from build123d import *

# Parameters (mm, degrees)
F0_R     = 1.5
F1_DEPTH = 2
F0_W     = 15.1
F0_H     = 20
F2_DEPTH = 7.7
F3_R     = 1


with BuildPart() as f1:
    # F0 (on Top) → F1 (new body)
    with BuildSketch(Plane.XY):
        with BuildLine():
            Line((-7.55, 10), (7.55, 10))
            Line((7.55, 10), (5.552786, 13.994427))
            ThreePointArc((5.552786, 13.994427), (4.815394, 14.801302), (3.763932, 15.1))
            Line((3.763932, 15.1), (-3.763932, 15.1))
            ThreePointArc((-3.763932, 15.1), (-4.815394, 14.801302), (-5.552786, 13.994427))
            Line((-5.552786, 13.994427), (-7.55, 10))
        make_face()
        with Locations((0, 12)):
            Circle(F0_R, mode=Mode.SUBTRACT)
    extrude(amount=F1_DEPTH)

    # F0 (on Top) → F2 (join)
    with BuildSketch(Plane.XY):
        Rectangle(F0_W, F0_H)
    extrude(amount=F2_DEPTH)

    # F3
    f3_edges = [f1.edges().sort_by_distance(p)[0] for p in [
        (0, -10, 7.7),
        (7.55, 0, 7.7),
        (0, 10, 7.7),
        (-7.55, 0, 7.7),
    ]]
    fillet(f3_edges, radius=F3_R)


solid = f1.part
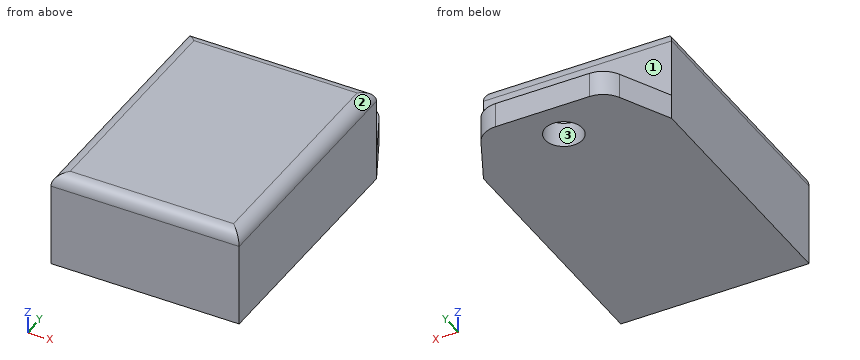
The listing builds one solid part. Answer for the finished solid, in the listing's coordinates (mm). Face numbers are marked on the shaded views. Coordinates: 2 decimals unless noted, no trailing zeros. Loops run counter-clockwise (first coordinate to the right, second up) from the corner with the lowest first, then second, coordinate; pieces in that order, holes last.
1) Find section C-C on z = 1. Write down the section's boundary in (x, y), then the cut area to 3 significant figures.
2) Determine the mould class of the marked faces 1, 2 and 3 for opening direction X: pulls with the +X half, pulls with the -X half, needs draft (parallel to the pull), parting line crosses it, or undercut.
3) Find section A-A on y = 12. Write down the section's boundary in (x, z).
4) Find section B-B on x = 0. Write down the section's boundary in (y, z).
5) Find the intervals of material crossed by L1, parallel to Y at x = 0, z = 1.3; L2, parallel to Z at x = 2.5, y = 11; L3, parallel to Y at x = 5.5, z = 5, in increasing order.
6) A flat-ended cylindrical pin translates along its axis: pin 1 Ø1.4 at (x, z) = (-3, 3.5) entering from +Y. Find the tip coordinate at first contact, or state that the pin passes through.
7) Find section D-D on x = 3. Write down the section's boundary in (y, z).
Values:
1. outline: (-7.55, -10) - (7.55, -10) - (7.55, 10) - (5.55, 13.99) arc R2 ccw to (3.76, 15.1) - (-3.76, 15.1) arc R2 ccw to (-5.55, 13.99) - (-7.55, 10) - close; hole circle Ø3 at (0, 12)
1. area: 358 mm2
2. face 1: needs draft
2. face 2: pulls with the +X half
2. face 3: undercut
3. outline: (-6.55, 0) - (-1.5, 0) - (-1.5, 2) - (-6.55, 2) - close; (1.5, 0) - (6.55, 0) - (6.55, 2) - (1.5, 2) - close
4. outline: (-10, 0) - (10.5, 0) - (10.5, 2) - (10, 2) - (10, 6.7) arc R1 ccw to (9, 7.7) - (-9, 7.7) arc R1 ccw to (-10, 6.7) - close; (13.5, 0) - (15.1, 0) - (15.1, 2) - (13.5, 2) - close
5. L1: y = -10 to 10.5, 13.5 to 15.1
5. L2: z = 0 to 2
5. L3: y = -10 to 10
6. pin 1: stops at y = 10
7. outline: (-10, 0) - (15.1, 0) - (15.1, 2) - (10, 2) - (10, 6.7) arc R1 ccw to (9, 7.7) - (-9, 7.7) arc R1 ccw to (-10, 6.7) - close
